Can you work these out from the model? Positions are in its coordinate system, mm. A direction names the side the tool comes from. Give positions to 0.01 mm unless a question says otherwise; leave off trailing zeros. Write each loop counter-clockwise with the first axis right and the second up, starting at its lowest first coordinate (ties: lowest second). Pieces come first, ordered by that corner, then holes.
Autodesk Inventor part; units mm, degrees
ref_plane "YZ Plane" through (0, 0, 0) normal (1, 0, 0) x (0, 1, 0)
ref_plane "XZ Plane" through (0, 0, 0) normal (0, 1, 0) x (-1, 0, 0)
ref_plane "XY Plane" through (0, 0, 0) normal (0, 0, 1) x (1, 0, 0)
sketch "Sketch1" plane through (0, 0, 0) normal (0, 0, 1) x (1, 0, 0)
  line L0 (5, 5) -> (5, -5)
  line L1 (-5, -5) -> (-5, 5)
  line L2 (5, 5) -> (-5, 5)
  line L3 (5, -5) -> (-5, -5)
  point P0 (0, 0)
  dimension "d16" = 10
  dimension "d17" = 10
  dimension "d18" = 5
  dimension "d19" = 5
extrude "Extrusion1" add sketch "Sketch1" along normal blind 10
sketch "Sketch3" plane through (0, 0, 10) normal (0, 0, 1) x (1, 0, 0)
  circle A0 centre (0, 0) radius 3.2
  dimension "d13" = 6.4
extrude "Extrusion3" cut sketch "Sketch3" against normal up to next
sketch "Sketch4" plane through (0, 0, 10) normal (0, 0, 1) x (1, 0, 0)
  arc A0 (-2.5, -7.0711) -> (2.5, -7.0711) centre (0, 0) ccw
  arc A1 (2.5, 7.0711) -> (-2.5, 7.0711) centre (0, 0) ccw
  line L0 (5, 5) -> (-5, 5)
  line L1 (-5, -5) -> (5, -5)
  line L2 (-2.5, 5) -> (2.5, 5)
  line L3 (2.5, -5) -> (-2.5, -5)
  line L4 (-2.5, 7.0711) -> (-2.5, 5)
  line L5 (-2.5, -5) -> (-2.5, -7.0711)
  line L6 (2.5, -7.0711) -> (2.5, -5)
  line L7 (2.5, 5) -> (2.5, 7.0711)
extrude "Extrusion4" add sketch "Sketch4" against normal blind 15
properties part number "PotHandle"
1) Suppose I cut it at B-B on y = -2.5. Write out the boundary of the cut face in (x, z).
Values follow:
outline: (-5, 0) - (-2, 0) - (-2, 10) - (-5, 10) - close; (2, 0) - (5, 0) - (5, 10) - (2, 10) - close
2) For faces 1 (the face through (4, 5, 5)), 2 (the face through (2.5, -6, 3)), 3 (the face through (-4, -5, 5)), which set-ups out of +Z, -Z, +X, -X, +Y, -Y let a thin tool reach every point of the face, with its end or its side?
Values follow:
face 1: +Z, -Z, +X, +Y
face 2: +Z, -Z, +X, -Y
face 3: +Z, -Z, -X, -Y
3) Suppose I cut it at D-D on x = 2.75. Write out the boundary of the cut face in (y, z).
Values follow:
outline: (-5, 0) - (-1.64, 0) - (-1.64, 10) - (-5, 10) - close; (1.64, 0) - (5, 0) - (5, 10) - (1.64, 10) - close
4) If we mould it in two halves opening along Y, with no side actions, what happens to faces 4 (the face through (-0.1, 3.4, 0)), 5 (the face through (0, -5, -2)), 6 (the face through (4, -5, 5)), 7 (the face through (-4, 5, 5))? For each: +Y half, -Y half, draft (parallel to the pull), parting line (faces both ways), or undercut.
Values follow:
face 4: undercut
face 5: undercut
face 6: -Y half
face 7: +Y half
5) Please list where these lines run through material, in increasing order: L1, parallel to Y at x = 0.25, z = -0.5; L2, parallel to Y at x = 0, z = 4; L3, parallel to Z at x = -4.5, y = -0.5.
Values follow:
L1: y = -7.5 to -5, 5 to 7.5
L2: y = -7.5 to -3.2, 3.2 to 7.5
L3: z = 0 to 10
6) Suppose I cut it at C-C on z = 1.25. Write out the boundary of the cut face in (x, y).
Values follow:
outline: (-5, -5) - (-2.5, -5) - (-2.5, -7.07) arc R7.5 ccw to (2.5, -7.07) - (2.5, -5) - (5, -5) - (5, 5) - (2.5, 5) - (2.5, 7.07) arc R7.5 ccw to (-2.5, 7.07) - (-2.5, 5) - (-5, 5) - close; hole circle Ø6.4 at (0, 0)
7) For pin 1 Ø5 at (x, z) = (-0.5, 7) entering from +Y; pin 2 Ø0.6 at (y, z) = (-6, 5) entering from -X; pin 3 Ø3 at (x, y) = (-2, -2.5) entering from -Z; pin 4 Ø1.2 at (x, z) = (-4, 4) entering from +Y, each with a flat end and sliding along its axis, tell me the tip position at first contact or that it passes through.
Values follow:
pin 1: stops at y = 7.5
pin 2: stops at x = -2.5
pin 3: stops at z = 0
pin 4: stops at y = 5
8) Suppose I cut it at A-A on x = 0. Write out the boundary of the cut face in (y, z).
Values follow:
outline: (-7.5, -5) - (-5, -5) - (-5, 0) - (-3.2, 0) - (-3.2, 10) - (-7.5, 10) - close; (3.2, 0) - (5, 0) - (5, -5) - (7.5, -5) - (7.5, 10) - (3.2, 10) - close
